Source: CAD feature listing. Evaluate the final solid. Frame: model axes, mm. Face numbers are marked on the shaded views. A direction names the side the tool comes from. Round coordinates to 2 decimals unless told otherwise and drop trailing zeros. Loops run counter-clockwise (first coordinate to the right, second up) from the corner with the lowest first, then second, coordinate; pieces in that order, holes last. Notation, with made-up numbers: (82, 36.5) - (98, 36.5) arc R34 cw to (98, 68.5) - close; hole circle Ø9 at (46.5, 81). An arc over 180 degrees is marked (long way). One line per question, with ' | ' between items.
from build123d import *

# Parameters (mm, degrees)
F0_W     = 25.4
F0_H     = 48.26
F1_DEPTH = 15.24
F2_R     = 3.175
F2_R_2   = 2.54
F3_DEPTH = 3.81
F5_DEPTH = 3.81


with BuildPart() as f1:
    # F0 (on Top) → F1 (new body)
    with BuildSketch(Plane.XY):
        with Locations((12.7, 24.13)):
            Rectangle(F0_W, F0_H)
    extrude(amount=F1_DEPTH)

    # F2 (on face) → F3 (join)
    with BuildSketch(Plane.XZ):
        with Locations((6.349094, 7.727245)):
            Circle(F2_R)
        with Locations((6.349094, 7.727245)):
            Circle(F2_R_2, mode=Mode.SUBTRACT)
    extrude(amount=F3_DEPTH)

    # F4 (on face) → F5 (join)
    with BuildSketch(Plane.XZ):
        Polygon((23.473546, 7.62), (21.261773, 11.450903), (16.838227, 11.450903), (14.626454, 7.62), (16.838227, 3.789097), (21.261773, 3.789097), align=None)
        Polygon((22.716174, 7.62), (20.883087, 4.445), (17.216913, 4.445), (15.383826, 7.62), (17.216913, 10.795), (20.883087, 10.795), align=None, mode=Mode.SUBTRACT)
    extrude(amount=F5_DEPTH)


solid = f1.part
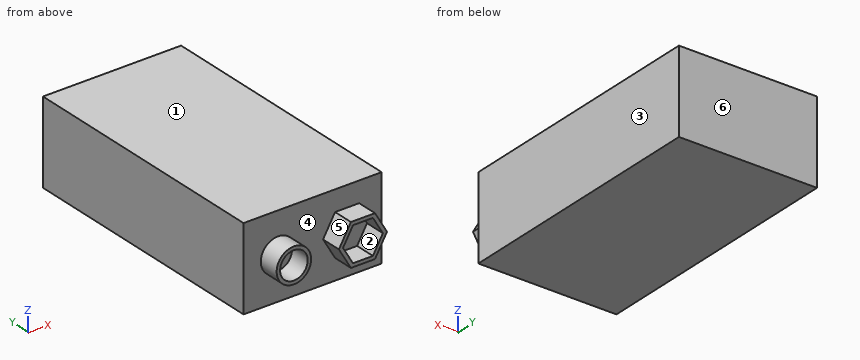
1. Section query A-A, the plane x = 18.5. Return loops of the section in (y, z) (3 decimals).
Worked out:
outline: (-3.81, 3.789) - (0, 3.789) - (0, 0) - (48.26, 0) - (48.26, 15.24) - (0, 15.24) - (0, 11.451) - (-3.81, 11.451) - (-3.81, 10.795) - (0, 10.795) - (0, 4.445) - (-3.81, 4.445) - close
2. Mould query, pull axis X, two halves, no side actions, for the marked faces 1, 2 and 3. Classes: released by +X, released by -X, zero draft, split by the parting line, or undercut.
Worked out:
face 1: zero draft | face 2: undercut | face 3: released by +X
3. Section query D-D, the plane z = 2.5. Return loops of the section in (x, y).
Worked out:
outline: (0, 0) - (25.4, 0) - (25.4, 48.26) - (0, 48.26) - close
4. Contact query for flat-ended pins moving along their axis: P1, Ø1.5, axis at x = 6, z = 8.5, coming from the -Y side; P2, Ø1.1, axis at x = 19.5, y = -2, coming from the -Z side. Output: stop coordinate, or through.
Worked out:
P1: stops at y = 0 | P2: stops at z = 3.79
5. Section query B-B, the plane z = 6.75. Return loops of the section in (x, y).
Worked out:
outline: (0, 0) - (3.33, 0) - (3.33, -3.81) - (4, -3.81) - (4, 0) - (8.69, 0) - (8.69, -3.81) - (9.37, -3.81) - (9.37, 0) - (15.13, 0) - (15.13, -3.81) - (15.89, -3.81) - (15.89, 0) - (22.21, 0) - (22.21, -3.81) - (22.97, -3.81) - (22.97, 0) - (25.4, 0) - (25.4, 48.26) - (0, 48.26) - close
6. Section query C-C, the plane x = 4.5. Return loops of the section in (y, z), plus the area to 3 significant figures.
Worked out:
outline: (-3.81, 5.15) - (0, 5.15) - (0, 0) - (48.26, 0) - (48.26, 15.24) - (0, 15.24) - (0, 10.31) - (-3.81, 10.31) - (-3.81, 9.47) - (0, 9.47) - (0, 5.99) - (-3.81, 5.99) - close | area: 742 mm2
7. Material intervals for probe 1 along Y at (x, z) = (17.5, 6); probe 2 along Z at (x, y) = (17, -1), sorted ascending.
Worked out:
probe 1: y = 0 to 48.26 | probe 2: z = 3.79 to 4.82, 10.42 to 11.45
8. Access query for the marked faces 4, 5 and 6. Directions: +Z, -Z, +X, -X, +Y, -Y. A direction counts if a zero-diameter tool reaches every point of the face in a straight line with its end or side. Return the directions, or none.
Worked out:
face 4: -Y | face 5: +Z, -Y | face 6: +Z, -Z, +X, -X, +Y
